Autodesk Fusion 360 part; units mm, degrees
sketch "Sketch1" plane through (0, 0, 0) normal (1, 0, 0) x (0, 1, 0)
  line L0 (3.44, 4.5007) -> (-3.44, 4.5007)
  line L1 (2.3572, -10.2) -> (2.3572, -8)
  line L2 (5.2993, 8) -> (5.2993, 6.6428)
  line L3 (-8.2, 5.4993) -> (-6.56, 5.4993)
  line L4 (4.7007, 3.3572) -> (6.6428, 5.2993)
  line L5 (5.2993, -6.6428) -> (5.2993, -8)
  line L6 (-8.2, -5.4993) -> (-8.2, -2.84)
  line L7 (-5.4993, -6.56) -> (-3.44, -4.5007)
  line L8 (-3.3572, 4.7007) -> (-5.2993, 6.6428)
  line L9 (8, 2.3572) -> (10.2, 4.5572)
  line L10 (10, -10) -> (10, -4.64)
  line L11 (10.2, -2.3572) -> (8, -2.3572)
  line L12 (5.4993, 6.56) -> (3.44, 4.5007)
  line L13 (8.2, 2.84) -> (10, 4.64)
  line L14 (-5.2993, 6.6428) -> (-5.2993, 8)
  line L15 (-8.2, 2.84) -> (-8.2, 5.4993)
  line L16 (-6.6428, -5.2993) -> (-8, -5.2993)
  line L17 (-10, 4.64) -> (-8.2, 2.84)
  line L18 (10.2, 10.2) -> (4.5572, 10.2)
  line L19 (-4.5572, 10.2) -> (-10.2, 10.2)
  line L20 (3.3572, 4.7007) -> (-3.3572, 4.7007)
  line L21 (-10.2, 2.3572) -> (-10.2, 4.5572)
  line L22 (10, 4.64) -> (10, 10)
  line L23 (-2.3572, 10.2) -> (-2.3572, 8)
  line L24 (-8, 2.3572) -> (-10.2, 2.3572)
  line L25 (-2.3572, 8) -> (-4.5572, 10.2)
  line L26 (6.56, 5.4993) -> (8.2, 5.4993)
  line L27 (-2.84, -8.2) -> (-5.4993, -8.2)
  line L28 (8, 2.3572) -> (10.2, 2.3572)
  line L29 (4.5007, 3.44) -> (6.56, 5.4993)
  line L30 (2.3572, -8) -> (4.5572, -10.2)
  line L31 (10.2, 2.3572) -> (10.2, 4.5572)
  line L32 (2.84, 8.2) -> (5.4993, 8.2)
  line L33 (4.64, 10) -> (2.84, 8.2)
  line L34 (4.5572, 10.2) -> (2.3572, 8)
  line L35 (10.2, -4.5572) -> (10.2, -2.3572)
  line L36 (10, -4.64) -> (8.2, -2.84)
  line L37 (10.2, -10.2) -> (10.2, -4.5572)
  line L38 (-3.3572, -4.7007) -> (3.3572, -4.7007)
  line L39 (-3.44, -4.5007) -> (3.44, -4.5007)
  line L40 (5.4993, -8.2) -> (2.84, -8.2)
  line L41 (5.4993, -6.56) -> (5.4993, -8.2)
  line L42 (8, -5.2993) -> (6.6428, -5.2993)
  line L43 (4.7007, -3.3572) -> (4.7007, 3.3572)
  line L44 (6.6428, -5.2993) -> (4.7007, -3.3572)
  line L45 (5.2993, -8) -> (2.3572, -8)
  line L46 (4.5572, -10.2) -> (10.2, -10.2)
  circle A0 centre (0, 0) radius 2.5
  line L47 (-15, 15) -> (15, -15) construction
  line L48 (10.2, -4.5572) -> (8, -2.3572)
  line L49 (8.2, -5.4993) -> (6.56, -5.4993)
  line L50 (4.5007, -3.44) -> (4.5007, 3.44)
  line L51 (15, -15) -> (15, 15)
  line L52 (8.2, -2.84) -> (8.2, -5.4993)
  line L53 (4.5572, -10.2) -> (2.3572, -10.2)
  line L54 (-15, -15) -> (15, -15)
  line L55 (15, 15) -> (-15, 15)
  line L56 (4.64, -10) -> (10, -10)
  line L57 (6.56, -5.4993) -> (4.5007, -3.44)
  line L58 (-15, 15) -> (-15, -15)
  line L59 (3.3572, -4.7007) -> (5.2993, -6.6428)
  line L60 (2.84, -8.2) -> (4.64, -10)
  line L61 (8, -2.3572) -> (8, -5.2993)
  line L62 (3.44, -4.5007) -> (5.4993, -6.56)
  line L63 (15, 15) -> (-15, -15) construction
  line L64 (-8.2, -2.84) -> (-10, -4.64)
  line L65 (-8, 5.2993) -> (-6.6428, 5.2993)
  line L66 (-8, -5.2993) -> (-8, -2.3572)
  line L67 (-3.44, 4.5007) -> (-5.4993, 6.56)
  line L68 (-5.4993, -8.2) -> (-5.4993, -6.56)
  line L69 (-4.5007, 3.44) -> (-4.5007, -3.44)
  line L70 (-5.4993, 6.56) -> (-5.4993, 8.2)
  line L71 (-10, -4.64) -> (-10, -10)
  line L72 (-10.2, 4.5572) -> (-8, 2.3572)
  line L73 (10.2, 4.5572) -> (10.2, 10.2)
  line L74 (8, 5.2993) -> (8, 2.3572)
  line L75 (2.3572, 8) -> (5.2993, 8)
  line L76 (-8, -2.3572) -> (-10.2, -4.5572)
  line L77 (-5.2993, -6.6428) -> (-3.3572, -4.7007)
  line L78 (-4.5572, -10.2) -> (-2.3572, -8)
  line L79 (-8, -2.3572) -> (-10.2, -2.3572)
  line L80 (5.4993, 8.2) -> (5.4993, 6.56)
  line L81 (-2.3572, -10.2) -> (-4.5572, -10.2)
  line L82 (-2.84, 8.2) -> (-4.64, 10)
  line L83 (-10, -10) -> (-4.64, -10)
  line L84 (-8, 2.3572) -> (-8, 5.2993)
  line L85 (2.3572, 10.2) -> (4.5572, 10.2)
  line L86 (8.2, 5.4993) -> (8.2, 2.84)
  line L87 (-10, 10) -> (-10, 4.64)
  line L88 (-5.2993, 8) -> (-2.3572, 8)
  line L89 (-10.2, -2.3572) -> (-10.2, -4.5572)
  line L90 (-10.2, -4.5572) -> (-10.2, -10.2)
  line L91 (-6.56, -5.4993) -> (-8.2, -5.4993)
  line L92 (-4.64, 10) -> (-10, 10)
  line L93 (-5.4993, 8.2) -> (-2.84, 8.2)
  line L94 (-6.56, 5.4993) -> (-4.5007, 3.44)
  line L95 (-2.3572, -8) -> (-2.3572, -10.2)
  line L96 (-4.5007, -3.44) -> (-6.56, -5.4993)
  line L97 (-4.64, -10) -> (-2.84, -8.2)
  line L98 (-10.2, -10.2) -> (-4.5572, -10.2)
  line L99 (-5.2993, -8) -> (-5.2993, -6.6428)
  line L100 (6.6428, 5.2993) -> (8, 5.2993)
  line L101 (5.2993, 6.6428) -> (3.3572, 4.7007)
  line L102 (-2.3572, -8) -> (-5.2993, -8)
  line L103 (10, 10) -> (4.64, 10)
  line L104 (-6.6428, 5.2993) -> (-4.7007, 3.3572)
  line L105 (-4.7007, -3.3572) -> (-6.6428, -5.2993)
  line L106 (-4.5572, 10.2) -> (-2.3572, 10.2)
  line L107 (-4.7007, 3.3572) -> (-4.7007, -3.3572)
  line L108 (2.3572, 8) -> (2.3572, 10.2)
  line L109 (-10.2, 10.2) -> (-10.2, 4.5572)
  line L110 (0, 15) -> (66, 15)
  line L111 (66, 15) -> (66, 10)
  line L112 (66, 10) -> (15, 10)
  line L113 (0, 15) -> (-66, 15)
  line L114 (-66, 15) -> (-66, 10)
  line L115 (-66, 10) -> (-15, 10)
  line L116 (66, 15) -> (76, 15)
  line L117 (76, 15) -> (76, 10)
  line L118 (76, 10) -> (66, 10)
  line L119 (66, 10) -> (66, 15)
  line L120 (-66, 15) -> (-76, 15)
  line L121 (-76, 15) -> (-76, 10)
  line L122 (-76, 10) -> (-66, 10)
  line L123 (-66, 10) -> (-66, 15)
  line L124 (-2.3572, -10.2) -> (2.3572, -10.2)
  line L125 (0, -10.2) -> (0, -15)
  dimension "d143" = 0.2
  dimension "d2" = 30
  dimension "d3" = 30
  dimension "d13" = 5
  dimension "d5" = 66
  dimension "d6" = 5
  dimension "d7" = 66
  dimension "d8" = 5
  dimension "d9" = 10
  dimension "d10" = 5
  dimension "d11" = 10
  dimension "d12" = 5
extrude "Extrude1" add sketch "Sketch1" along normal mid plane 20 contours L1 L5 L38 L45 L59 L77 L95 L99 L102 L124 | L51 L54 L55 L58 L110 L113 | L58 L113 L114 L115 L123 | L51 L110 L111 L112 L119 | L114 L120 L121 L122 L123 | L111 L116 L117 L118 L119
extrude "Extrude2" cut sketch "Sketch1" along normal mid plane 15 contours L1 L5 L38 L45 L59 L77 L95 L99 L102 L124
sketch "Sketch2" plane through (0, 0, -15) normal (0, 0, -1) x (1, 0, 0)
  line L0 (-10, -15) -> (10, -15)
  line L1 (10, -15) -> (10, 15)
  line L2 (10, 15) -> (-10, 15)
  line L3 (-10, 15) -> (-10, -15)
  circle A0 centre (0, 0) radius 2.5
  dimension "d18" = 5
extrude "Extrude3" cut sketch "Sketch2" against normal blind 17 contours A0
sketch "Sketch3" plane through (0, 0, 15) normal (0, 0, 1) x (-1, 0, 0)
  line L0 (10, 76) -> (-10, 76)
  line L1 (-10, 76) -> (-10, -76)
  line L2 (-10, -76) -> (10, -76)
  line L3 (10, -76) -> (10, 76)
  circle A0 centre (0, 66) radius 2
  line L4 (0, 66) -> (0, 76)
  circle A1 centre (0, -66) radius 2
  line L5 (-10, 76) -> (10, 76)
  line L6 (10, 76) -> (10, 75)
  line L7 (10, 75) -> (-10, 75)
  line L8 (-10, 75) -> (-10, 76)
  line L9 (-10, -76) -> (10, -76)
  line L10 (10, -76) -> (10, -75)
  line L11 (10, -75) -> (-10, -75)
  line L12 (-10, -75) -> (-10, -76)
  point P0 (0, -66)
  dimension "d21" = 4
  dimension "d22" = 4
  dimension "d25" = 1
  dimension "d26" = 20
  dimension "d27" = 1
extrude "Extrude4" cut sketch "Sketch3" against normal blind 20 contours A0 | A1
fillet "Fillet2" radius 2 2 edges at (0, 76, 10) (0, -76, 10)
fillet "Fillet3" radius 20 2 edges at (0, -15, 10) (0, 15, 10)
fillet "Fillet4" radius 5 2 edges at (0, 15, -15) (0, -15, -15)
equation "d5 = ( 132 / 2 ) * 1 mm"
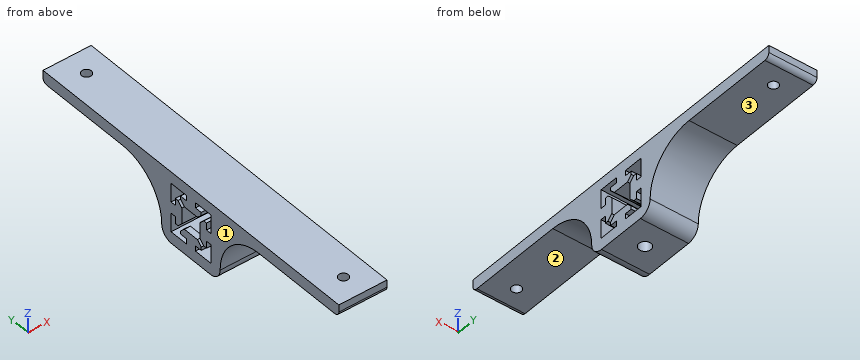
The model under review builds one solid part; all positions refer to its coordinate system, in mm. Face numbers are marked on the shaded views. A direction names the side the tool comes from. Coordinates: 2 decimals unless noted, no trailing zeros. Loops run counter-clockwise (first coordinate to the right, second up) from the corner with the lowest first, then second, coordinate; pieces in that order, holes last. Notation, with made-up numbers: (3, 10.25) -> (61, 10.25) arc R22 ccw to (61, 39.25) -> close; hole circle Ø10 at (-29.5, 86.25). An arc over 180 degrees is marked (long way). Use a Markdown table: item, result. Add a question column.
1. Add section B-B on z = -1. Write out the cut boundary in (x, y).
2. Add section A-A on y = -66. Write out the cut boundary in (x, z), plus the area to 3 significant figures.
3. Add section C-C on y = 25.5. Write out the cut boundary in (x, z).
4. To check wall thickness, follow line 1 (Z direction, x = 6, y = 7.5); line 2 (Y direction, x = 0, z = 12.5); line 3 (X direction, y = -66, z = 12.35). State the ranges of each line that lie inside material, in increasing order.
5. Clearance check with flat-ended pins moving along their axes: pin 1 Ø6.5 at (x, z) = (4.5, 7.5) entering from -Y; pin 2 Ø1.1 at (x, z) = (-8, -7.5) entering from -Y; pin 3 Ø1.1 at (x, z) = (-3.5, 7) entering from -Y. State where each tip first meets the part, or that it passes through.
6. Add section D-D on y = -31.5. Write out the cut boundary in (x, z).
7. Machinability: for the marked faces 1, 2 and 3, which of the approach directions +Z, -Z, +X, -X, +Y, -Y give a long, thin tool a straight path to every point of the face, cutting with its end or side? Answer none if there is none.
Returned:
| question | item | result |
|---|---|---|
| 1 | outline | (-10, -17.14) -> (10, -17.14) -> (10, -4.7) -> (-10, -4.7) -> close; (-10, 4.7) -> (10, 4.7) -> (10, 17.14) -> (-10, 17.14) -> close |
| 2 | outline | (-10, 10) -> (-2, 10) -> (-2, 15) -> (-10, 15) -> close; (2, 10) -> (10, 10) -> (10, 15) -> (2, 15) -> close |
| 2 | area | 80.0 mm² |
| 3 | outline | (-10, 7.6) -> (10, 7.6) -> (10, 15) -> (-10, 15) -> close |
| 4 | line 1 | z = -15 to -10.2, -5.3 to 5.3, 10.2 to 15 |
| 4 | line 2 | y = -76 to -68, -64 to 64, 68 to 76 |
| 4 | line 3 | x = -10 to -2, 2 to 10 |
| 5 | pin 1 | stops at y = -75.56 |
| 5 | pin 2 | stops at y = -15.23 |
| 5 | pin 3 | stops at y = -25.41 |
| 6 | outline | (-10, 9.69) -> (10, 9.69) -> (10, 15) -> (-10, 15) -> close |
| 7 | face 1 | +Z, -Z, -X, +Y, -Y |
| 7 | face 2 | -Z, +X, -X, -Y |
| 7 | face 3 | -Z, +X, -X, +Y |
